Design review of the part built by this model. Coordinates are the model's own, in mm. A direction names the side the tool comes from. Round coordinates to 2 decimals unless told otherwise and drop trailing zeros. Loops run counter-clockwise (first coordinate to the right, second up) from the corner with the lowest first, then second, coordinate; pieces in that order, holes last. Notation, with made-up numbers: (-2, 35) -> (13, 35) arc R32 cw to (13, 68) -> close; hole circle Ø8 at (42.25, -3). An arc over 180 degrees is marked (long way). Answer as CSV lines item,"result". Start each with the question number.
(1) Take a section at C-C, the plane z = 0.75. State how many separate pieces and enclosed holes the cut face has, and give its area (3 significant figures).
(2) Machinability: for faces 4 (the face through (20.25, -6, 2)), 5 (the face through (-5, 17, 2)), 6 (the face through (14, 0, 2)), 7 (the face through (23.25, -6, 2)), 8 (the face through (0, 8, 4)), which of the approach directions +Z, -Z, +X, -X, +Y, -Y give a long, thin tool a straight path to every point of the face, cutting with its end or side? Answer none if there is none.
(3) Take a section at B-B, the plane x = -14. Write out the cut boundary in (y, z).
(4) Draft analysis for pull direction X (two halves, no side actions). For faces 1 (the face through (-20.25, -6, 2)), 2 (the face through (-14, 0, 2)), 3 (the face through (5, 17, 2)), state which applies: +X half, -X half, draft (parallel to the pull), parting line (faces both ways), or undercut.
(5) Take a section at D-D, the plane x = -1. Write out the cut boundary in (y, z).
(6) To check wall thickness, follow line 1 (Y direction, x = 0, z = 2.4) (3 decimals); line 2 (Y direction, x = -18, z = 3); line 3 (Y direction, x = 0.5, z = 1.4). State the ranges of each line that lie inside material, in increasing order. Write a range as from..to.
(7) Take a section at A-A, the plane y = -4. Write out the cut boundary in (x, z).
(8) For P1, Ø1.5, axis at y = 12, z = 1.5, coming from the +X side; P2, Ø2, axis at x = 17.5, z = 2.5, coming from the +Y side; P3, Ø10, axis at x = 14, y = 34.5, coming from the +Z side; P4, Ø2, axis at y = 10, z = 2.5, coming from the -X side, all flat-tipped, find the tip position at first contact; note any pin that passes through.
from build123d import *

# Parameters (mm, degrees)
F0_W     = 3
F0_H     = 3
F0_W_2   = 40.5
F0_H_2   = 6.25
F0_W_3   = 10
F0_H_3   = 40
F1_DEPTH = 4
F2_R     = 4.99999
F3_R     = 2.375
F4_DEPTH = 4.001


# Not quite as in the source:
# - a fillet or chamfer is up to 0.001 mm smaller than in the source, because OpenCascade refuses the exact size


with BuildPart() as f1:
    # F0 (on Top) → F1 (new body)
    with BuildSketch(Plane.XY):
        with Locations((21.75, -1.5)):
            Rectangle(F0_W, F0_H)
        Polygon((20.25, -3), (20.25, 0), (5, 0), (-5, 0), (-23.25, 0), (-23.25, -12.25), (23.25, -12.25), (23.25, -3), align=None)
        with Locations((0, -6.125)):
            Rectangle(F0_W_2, F0_H_2, mode=Mode.SUBTRACT)
        with Locations((0, 20)):
            Rectangle(F0_W_3, F0_H_3)
    extrude(amount=F1_DEPTH)

    # F2 (radius 5 in the source; OpenCascade refuses exactly that, so slightly less here)
    f2_edges = [f1.edges().sort_by_distance(p)[0] for p in [
        (5, 40, 2),
        (-5, 40, 2),
    ]]
    fillet(f2_edges, radius=F2_R)

    # F3 (on face) → F4 (cut, through all)
    with BuildSketch(Plane.XY.offset(4)):
        with Locations((0, 35)):
            Circle(F3_R)
    extrude(amount=-F4_DEPTH, mode=Mode.SUBTRACT)


solid = f1.part
The answers:
1,separate pieces,"1"
1,enclosed holes,"2"
1,area,"688 mm²"
2,face 4,"+Z, -Z"
2,face 5,"+Z, -Z, -X, +Y"
2,face 6,"+Z, -Z, +X, +Y"
2,face 7,"+Z, -Z, +X, +Y, -Y"
2,face 8,"+Z, +X, -X, +Y, -Y"
3,outline,"(-12.25, 0) -> (-9.25, 0) -> (-9.25, 4) -> (-12.25, 4) -> close; (-3, 0) -> (0, 0) -> (0, 4) -> (-3, 4) -> close"
4,face 1,"undercut"
4,face 2,"draft"
4,face 3,"+X half"
5,outline,"(-12.25, 0) -> (-9.25, 0) -> (-9.25, 4) -> (-12.25, 4) -> close; (-3, 0) -> (32.85, 0) -> (32.85, 4) -> (-3, 4) -> close; (37.15, 0) -> (39.9, 0) -> (39.9, 4) -> (37.15, 4) -> close"
6,line 1,"-12.25..-9.25, -3..32.625, 37.375..40"
6,line 2,"-12.25..-9.25, -3..0"
6,line 3,"-12.25..-9.25, -3..32.68, 37.32..39.97"
7,outline,"(-23.25, 0) -> (-20.25, 0) -> (-20.25, 4) -> (-23.25, 4) -> close; (20.25, 0) -> (23.25, 0) -> (23.25, 4) -> (20.25, 4) -> close"
8,P1,"x = 5"
8,P2,"y = 0"
8,P3,"through"
8,P4,"x = -5"
